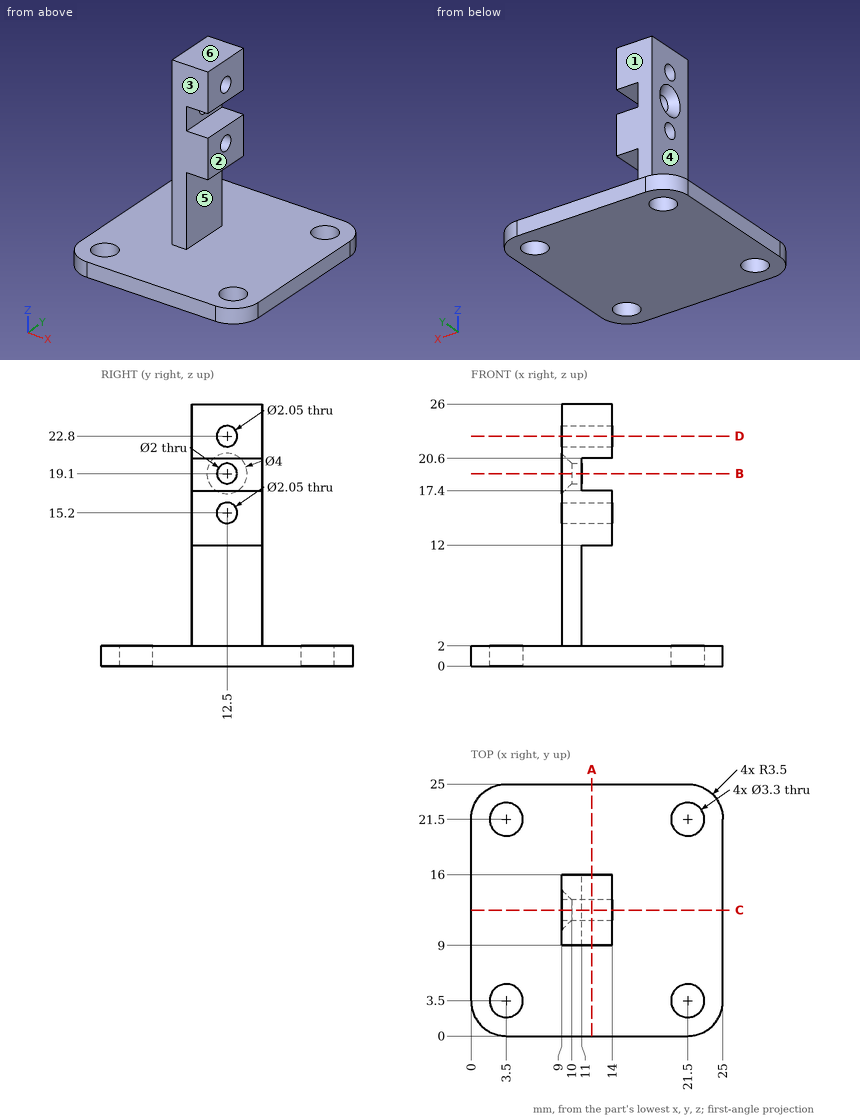
Part print with two shaded views. Sizes in mm from the minimum x, y, z corner. A direction names the side the tool comes from. Give positions to 0.01 mm unless a question says otherwise; leave off trailing zeros. Order: outer loops, then holes, each group sorted by start corner. A loop starts at its lowest first (then second) coordinate and runs counter-clockwise, first axis right, second up.
(1) Flat gauge pins, fed straight in: pin 1 (6 mm diameter, centred on y = 11, z = 24, fed in from +X); pin 2 (6 mm diameter, centred on x = 16, z = 10, fed in from -Y); pin 3 (1.5 mm diameter, centred on x = 9.5, z = 5, fed in from +Y); pin 4 (2.5 mm diameter, centred on x = 3.5, y = 21.5, fed in from -Z). Where does each tip first touch, or does it go through?
(2) Saw through at A-A, the plane x = 12. Give the cut face in (y, z) (3 decimals).
(3) Saw through at C-C, the plane y = 12.5. Give the cut face in (x, z) (3 decimals).
(4) Mould opens along Z. For the marked faces 4, 5 and 6 say: released by +Z, released by -Z, zero draft, split by the parting line, or undercut.
(5) Saw through at B-B, the plane z = 19.1. Give the cut face in (x, y), then the cut area to 3 significant figures.
(6) Tool access for the marked faces 1, 2 and 3: list every direction of +Z, -Z, +X, -X, +Y, -Y with a clear straight run to the whole face (end or side of a thin tool).
(7) Saw through at D-D, the plane z = 22.8. Give the cut face in (x, y) (3 decimals), then the cut area to 4 significant figures.
(8) Drill centre lines: L1, parallel to Y at x = 3.5, z = 1.05; L2, parallel to Z at x = 10.65, y = 12.5 (3 decimals); L3, parallel to Z at x = 11.9, y = 12.5 (3 decimals). Where is each one in solid material? Low to high.
Results found:
1. pin 1: stops at x = 14
1. pin 2: stops at y = 9
1. pin 3: stops at y = 16
1. pin 4: passes through
2. outline: (0, 0) - (25, 0) - (25, 2) - (0, 2) - close; (9, 12) - (16, 12) - (16, 17.4) - (9, 17.4) - close; (9, 20.6) - (16, 20.6) - (16, 26) - (9, 26) - close; hole circle Ø2.05 at (12.5, 15.2); hole circle Ø2.05 at (12.5, 22.8)
3. outline: (0, 0) - (25, 0) - (25, 2) - (11, 2) - (11, 12) - (14, 12) - (14, 14.175) - (9, 14.175) - (9, 2) - (0, 2) - close; (9, 16.225) - (14, 16.225) - (14, 17.4) - (11, 17.4) - (11, 18.1) - (10, 18.1) - (9, 17.1) - close; (9, 21.1) - (10, 20.1) - (11, 20.1) - (11, 20.6) - (14, 20.6) - (14, 21.775) - (9, 21.775) - close; (9, 23.825) - (14, 23.825) - (14, 26) - (9, 26) - close
4. face 4: zero draft
4. face 5: undercut
4. face 6: released by +Z
5. outline: (9, 9) - (11, 9) - (11, 11.5) - (10, 11.5) - (9, 10.5) - close; (9, 14.5) - (10, 13.5) - (11, 13.5) - (11, 16) - (9, 16) - close
5. area: 9.00 mm2
6. face 1: +Z, +X, -X, +Y
6. face 2: +Z, +X, +Y, -Y
6. face 3: +Z, +X, -X, -Y
7. outline: (9, 9) - (14, 9) - (14, 11.475) - (9, 11.475) - close; (9, 13.525) - (14, 13.525) - (14, 16) - (9, 16) - close
7. area: 24.75 mm2
8. L1: y = 0 to 1.85, 5.15 to 19.85, 23.15 to 25
8. L2: z = 0 to 14.175, 16.225 to 18.1, 20.1 to 21.775, 23.825 to 26
8. L3: z = 0 to 2, 12 to 14.175, 16.225 to 17.4, 20.6 to 21.775, 23.825 to 26
